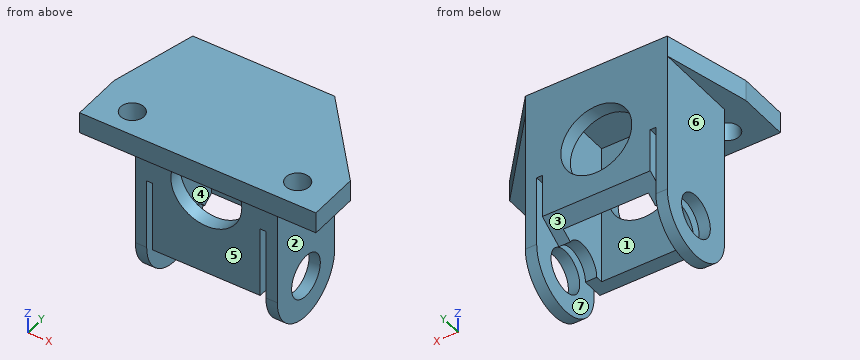
Autodesk Inventor part; units mm, degrees
ref_plane "Work Plane4" through (7.6, 2, 20) normal (-1, 0, 0) x (0, 0, 1)
ref_plane "YZ Plane" through (0, 0, 0) normal (1, 0, 0) x (0, 1, 0)
ref_plane "XZ Plane" through (0, 0, 0) normal (0, 1, 0) x (-1, 0, 0)
sketch "Sketch1" plane through (0, 0, 0) normal (0, 0, 1) x (1, 0, 0)
  line L0 (0, 0) -> (15.2, 0)
  line L1 (15.2, 0) -> (15.2, 12)
  line L2 (15.2, 12) -> (0, 12)
  line L3 (0, 12) -> (0, 0)
  line L4 (1.6, 10) -> (13.6, 10)
  line L5 (13.6, 10) -> (13.6, 2)
  line L6 (13.6, 2) -> (1.6, 2)
  line L7 (1.6, 2) -> (1.6, 10)
  dimension "d0" = 15.2
  dimension "d1" = 12
  dimension "d2" = 1.6
  dimension "d3" = 2
  dimension "d4" = 2
  dimension "d5" = 1.6
extrude "Extrusion1" add sketch "Sketch1" along normal blind 20
sketch "Sketch2" plane through (0, 0, 0) normal (1, 0, 0) x (0, 1, 0)
  line L0 (0, 0) -> (12, 0) construction
  line L1 (6, 13.0663) -> (6, -2.0093) construction
  line L2 (0, 0) -> (0, 20) construction
  line L3 (12, 0) -> (12, 20) construction
  line L4 (6, 0) -> (12, 3.8224)
  line L5 (12, 3.8224) -> (12, 0)
  line L6 (12, 0) -> (6, 0)
  dimension "d8" = 12
  dimension "d9" = 6
  dimension "d10" = 32.5
extrude "Extrusion2" cut sketch "Sketch2" along normal through all
sketch "Sketch9" plane through (0, 0, 20) normal (-1, 0, 0) x (0, 0, 1)
  line L0 (-20, 0) -> (0, 0) construction
  line L1 (0, 12) -> (0, 0) construction
  line L2 (-16.1776, 12) -> (0, 12) construction
  line L3 (-20, 0) -> (-20, 14.5103) construction
  line L4 (-20, 0) -> (0, 0)
  line L5 (0, 12) -> (0, 0)
  line L6 (0, 12) -> (-20, 12)
  arc A0 (-20, 12) -> (-20, 0) centre (-20, 6) ccw
extrude "Extrusion8" add sketch "Sketch9" along normal blind 2.4
sketch "Sketch4" plane through (1.6, 2, 20) normal (1, 0, 0) x (0, 0, -1)
  circle A0 centre (20, 4) radius 3
  point P0 (20, -2)
  dimension "d14" = 6
extrude "Extrusion3" cut sketch "Sketch4" along normal through all both and the other way through all
sketch "Sketch11" plane through (15.2, 12, 20) normal (0, 1, 0) x (1, 0, 0)
  line L0 (0, 0) -> (-17.6, 0) construction
  line L1 (-15.2, 26) -> (-15.2, 20) construction
  line L2 (-15.2, 26) -> (-16, 26)
  line L3 (-16, 26) -> (-16, 10)
  line L4 (-16, 10) -> (-15.2, 10)
  line L5 (-15.2, 10) -> (-15.2, 26)
  line L6 (-15.2, 20) -> (-13.6, 20) construction
  dimension "d38" = 10
  dimension "d39" = 0.8
extrude "Extrusion9" cut sketch "Sketch11" against normal through all
ref_plane "Work Plane4" through (7.6, 2, 20) normal (-1, 0, 0) x (0, 0, 1)
mirror "Mirror3" about plane through (7.6, 2, 20) normal (-1, 0, 0) of "Extrusion8", "Extrusion3", "Extrusion9"
sketch "Sketch14" plane through (0, 0, 20) normal (0, 0, 1) x (1, 0, 0)
  line L0 (17.6, 0) -> (-2.4, 0) construction
  line L1 (-2.4, 12) -> (17.6, 12) construction
  line L2 (-5.4, 0) -> (-5.4, -7.2)
  line L3 (-5.4, -7.2) -> (27.9, -7.2)
  line L4 (27.9, -7.2) -> (27.9, 0)
  line L5 (17.6, 12) -> (-2.4, 12)
  line L6 (-5.4, -3.6) -> (27.9, -3.6) construction
  circle A0 centre (-0.4, -3.6) radius 1.65
  line L7 (7.6, 12) -> (7.6, -12.1697) construction
  circle A1 centre (22.9, -3.6) radius 1.65
  line L8 (-5.4, 0) -> (-2.4, 12)
  line L9 (17.6, 12) -> (27.9, 0)
  point P0 (0, 0)
  dimension "d54" = 7.2
  dimension "d55" = 3.3
  dimension "d56" = 8
  dimension "d57" = 15.3
  dimension "d58" = 5
  dimension "d59" = 5
extrude "Extrusion12" add sketch "Sketch14" along normal blind 3
sketch "Sketch15" plane through (-2.4, 0, 0) normal (0, -1, 0) x (1, 0, 0)
  line L0 (2.4, 0) -> (17.6, 0) construction
  line L1 (17.6, 10) -> (18.4, 10) construction
  line L2 (10, 0) -> (10, 23.7385) construction
  circle A0 centre (10, 12) radius 5
  dimension "d62" = 10
  dimension "d63" = 12
extrude "Extrusion13" cut sketch "Sketch15" against normal through all
equation "\"d9\" = 0.5 * d8"
properties part number "chain_end_extruder"
Design review of the part built by this model. Coordinates are the model's own, in mm. Face numbers are marked on the shaded views. A direction names the side the tool comes from. Give positions to 0.01 mm unless a question says otherwise; leave off trailing zeros. Loops run counter-clockwise (first coordinate to the right, second up) from the corner with the lowest first, then second, coordinate; pieces in that order, holes last. Notation, with made-up numbers: M -7.5,26 L 43.5,26 A14 cw 43.5,49 Z; hole C -27.75,-28 d6. An arc over 180 degrees is marked long. Write item = value, one per line.
Q1. Insertion check: pin 1 (13 mm diameter, centred on x = 7.6, z = 12, fed in from -Y); pin 2 (5 mm diameter, centred on y = 3.5, z = 7.5, fed in from -X); pin 3 (4 mm diameter, centred on x = 9.5, y = 4.5, fed in from -Z). Each pin has a flat end and moves straight along its axis. Give the tip position at first contact, or say it passes through.
Output values:
pin_1 = 0
pin_2 = -2.4
pin_3 = 20
Q2. We need section A-A (z = 12). Give the boundary of the cut face in (x, y), plus the area to 3 significant figures.
Output values:
outline = M -2.4,0 L 2.6,0 L 2.6,2 L 1.6,2 L 1.6,10 L 2.6,10 L 2.6,12 L -2.4,12 Z; M 12.6,0 L 17.6,0 L 17.6,12 L 12.6,12 L 12.6,10 L 13.6,10 L 13.6,2 L 12.6,2 Z
area = 104 mm^2
Q3. For the marked faces 4, 5, 6 and 7, list the 3-axis set-ups (+Z, -Z, +X, -X, +Y, -Y) from which the entire face can be reached by the end or side of a thin tool; tool diameter is ignored.
Output values:
face_4 = -Z
face_5 = -Z, +X, -X, -Y
face_6 = -Z, -X, +Y, -Y
face_7 = -Z, +Y, -Y
Q4. We need section D-D (x = 22.9). Give the boundary of the cut face in (y, z).
Output values:
outline = M -7.2,20 L -5.25,20 L -5.25,23 L -7.2,23 Z; M -1.95,20 L 5.83,20 L 5.83,23 L -1.95,23 Z
Q5. We need section B-B (y = -3.6). Give the boundary of the cut face in (x, z).
Output values:
outline = M -5.4,20 L -2.05,20 L -2.05,23 L -5.4,23 Z; M 1.25,20 L 21.25,20 L 21.25,23 L 1.25,23 Z; M 24.55,20 L 27.9,20 L 27.9,23 L 24.55,23 Z
Q6. To check wall thickness, follow line 1 (X direction, y = 5, z = 6); line 2 (Y direction, x = 3.5, z = 18.5); line 3 (Z direction, x = 17, y = 6). State the ranges of each line that lie inside material, in increasing order. Write a range as [from, to].
Output values:
line_1 = [-2.4, -0.8], [0, 1.6], [13.6, 15.2], [16, 17.6]
line_2 = [0, 2], [10, 12]
line_3 = [-6, -3], [3, 23]
Q7. We need section C-C (x = 7). Give the boundary of the cut face in (y, z).
Output values:
outline = M -7.2,20 L 0,20 L 0,16.96 L 2,16.96 L 2,20 L 10,20 L 10,16.96 L 12,16.96 L 12,23 L -7.2,23 Z; M 0,0 L 2,0 L 2,7.04 L 0,7.04 Z; M 10,2.55 L 12,3.82 L 12,7.04 L 10,7.04 Z
Q8. Draft analysis for pull direction Y (two halves, no side actions). For the marked faces 1, 2 and 3, state which applies: +Y half, -Y half, draft (parallel to the pull), parting line (faces both ways), or undercut.
Output values:
face_1 = undercut
face_2 = draft
face_3 = +Y half
